Autodesk Inventor part; units mm, degrees
ref_plane "YZ Plane" through (0, 0, 0) normal (1, 0, 0) x (0, 1, 0)
ref_plane "XZ Plane" through (0, 0, 0) normal (0, 1, 0) x (-1, 0, 0)
ref_plane "XY Plane" through (0, 0, 0) normal (0, 0, 1) x (1, 0, 0)
sketch "スケッチ1" plane through (0, 0, 0) normal (0, 0, 1) x (1, 0, 0)
  circle A0 centre (-4.75, 48) radius 1.55
  circle A1 centre (4.75, 48) radius 1.55
  circle A2 centre (-4.75, -48) radius 1.55
  circle A3 centre (4.75, -48) radius 1.55
  line L0 (-4.75, -48) -> (4.75, -48) construction
  line L1 (4.75, -48) -> (4.75, 48) construction
  line L2 (4.75, 48) -> (-4.75, 48) construction
  line L3 (-4.75, 48) -> (-4.75, -48) construction
  line L4 (-4.75, -48) -> (4.75, 48) construction
  line L5 (4.75, -48) -> (-4.75, 48) construction
  line L6 (-17.75, 61) -> (50.25, 61)
  line L7 (50.25, 61) -> (50.25, -104)
  line L8 (50.25, -104) -> (-17.75, -104)
  line L9 (-17.75, -104) -> (-17.75, 61)
  circle A4 centre (44.25, 55) radius 1.55
  line L10 (16.25, 61) -> (16.25, -104) construction
  line L11 (16.25, -21.5) -> (50.25, -21.5) construction
  circle A5 centre (21.25, 55) radius 1.55
  circle A6 centre (33.25, 55) radius 1.55
  line L12 (16.25, 19.75) -> (50.25, 19.75) construction
  line L13 (16.25, 40.375) -> (50.25, 40.375) construction
  circle A7 centre (44.25, 25.75) radius 1.55
  circle A8 centre (44.25, -15.5) radius 1.55
  circle A9 centre (44.25, 13.75) radius 1.55
  circle A10 centre (44.25, -98) radius 1.55
  circle A11 centre (21.25, -98) radius 1.55
  circle A12 centre (33.25, -98) radius 1.55
  circle A13 centre (44.25, -68.75) radius 1.55
  circle A14 centre (44.25, -27.5) radius 1.55
  circle A15 centre (44.25, -56.75) radius 1.55
  circle A16 centre (-11.75, 55) radius 1.55
  circle A17 centre (11.25, 55) radius 1.55
  circle A18 centre (-0.75, 55) radius 1.55
  circle A19 centre (-11.75, 25.75) radius 1.55
  circle A20 centre (-11.75, -15.5) radius 1.55
  circle A21 centre (-11.75, 13.75) radius 1.55
  circle A22 centre (-11.75, -27.5) radius 1.55
  circle A23 centre (-11.75, -56.75) radius 1.55
  circle A24 centre (11.25, -98) radius 1.55
  circle A25 centre (-0.75, -98) radius 1.55
  circle A26 centre (-11.75, -98) radius 1.55
  circle A27 centre (-11.75, -68.75) radius 1.55
  circle A28 centre (-4.75, 38) radius 1.55
  circle A29 centre (4.75, 38) radius 1.55
  circle A30 centre (-4.75, -58) radius 1.55
  circle A31 centre (4.75, -58) radius 1.55
  circle A32 centre (-4.75, 28) radius 1.55
  circle A33 centre (4.75, 28) radius 1.55
  circle A34 centre (-4.75, -68) radius 1.55
  circle A35 centre (4.75, -68) radius 1.55
  circle A36 centre (-4.75, 18) radius 1.55
  circle A37 centre (4.75, 18) radius 1.55
  circle A38 centre (-4.75, -78) radius 1.55
  circle A39 centre (4.75, -78) radius 1.55
  circle A40 centre (-4.75, 8) radius 1.55
  circle A41 centre (4.75, 8) radius 1.55
  circle A42 centre (-4.75, -88) radius 1.55
  circle A43 centre (4.75, -88) radius 1.55
  circle A44 centre (25.5, 36.25) radius 10.75
  line L14 (14.75, 47) -> (36.25, 47) construction
  line L15 (36.25, 47) -> (36.25, -90) construction
  line L16 (36.25, -90) -> (14.75, -90) construction
  line L17 (14.75, -90) -> (14.75, 47) construction
  circle A45 centre (25.5, -0.75) radius 10.75
  circle A46 centre (25.5, -37.75) radius 10.75
  circle A47 centre (25.5, -74.75) radius 10.75
  circle A48 centre (4.75, 48) radius 2.75 construction
  point P0 (0, 0)
  dimension "d0" = 3.1
  dimension "d1" = 9.5
  dimension "d2" = 96
  dimension "d3" = 13
  dimension "d4" = 13
  dimension "d7" = 165
  dimension "d8" = 68
  dimension "d16" = 3.1
  dimension "d17" = 6
  dimension "d18" = 6
  dimension "d19" = 5
  dimension "d20" = 17
  dimension "d21" = 41.25
  dimension "d22" = 20.625
  dimension "d25" = 10
  dimension "d30" = 10
  dimension "d31" = 8
  dimension "d32" = 8
  dimension "d35" = 37
  dimension "d40" = 8
  dimension "d41" = 5.5
extrude "押し出し1" add sketch "スケッチ1" along normal blind 2
equation "\"d1\" = d20_1"
equation "\"d4\" = d3"
equation "\"d8\" = 足_短辺"
equation "\"d18\" = d17"
equation "\"d20\" = 0.25 * d8"
equation "\"d21\" = 0.25 * d7"
equation "\"d22\" = 0.5 * d21"
equation "\"d31\" = d32"
equation "\"d40\" = d31"
equation "\"H_head\" = 96"
equation "\"H_leg\" = 306"
equation "\"足の面積\" = 12720.125"
equation "\"現在の面積\" = 11560"
equation "\"足_短辺\" = 68"
equation "\"円柱\" = 313.5"
equation "\"胴体中心から手先\" = 342"
equation "\"H_leg_1\" = 186.2"
equation "\"H_leg_MAX\" = 399"
equation "\"H_head_1\" = 26.6"
equation "\"H_head_MAX\" = 142.5"
properties part number "足裏_メインフレーム_1_3" material "GFRP"
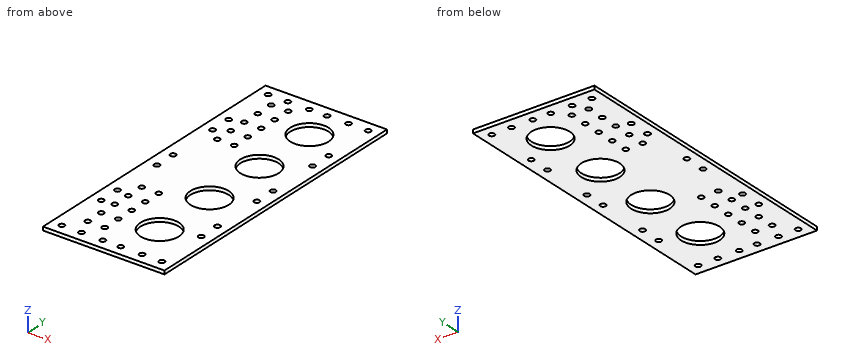
Build history of the part. All positions in model axes, mm. Give positions to 0.01 mm unless a question says otherwise; leave off trailing zeros. Loops run counter-clockwise (first coordinate to the right, second up) from the corner with the lowest first, then second, coordinate; pieces in that order, holes last. Notation, with made-up numbers: (23.25, 39.5) -> (57.25, 39.5) arc R22 cw to (57.25, 57.5) -> close; hole circle Ø3 at (5, 17.25). An arc over 180 degrees is marked (long way). One line per question, with ' | ' between items. Start each with the question number.
1) Cut at D-D (y = -0.75). Give the cut face in (x, z), plus the area to 3 significant figures.
2) Cut at C-C (x = 25.5). Give the cut face in (y, z), plus the area to 3 significant figures.
3) Cut at B-B (y = -98). Give the cut face in (x, z).
4) Cut at A-A (x = -0.75). Give the cut face in (y, z), plus the area to 3 significant figures.
5) Probe L1, parallel to X at y = -56, z = 1.6; L2, parallel to Y at x = 0, z = 0.9; L3, parallel to Y at x = 0.5, z = 1.75. List the from-to ranges inside material, lowest first.
6) Pin check, flat tips, straight feed: pin 1 (1.9 mm diameter, centred on x = 44.25, y = -98, fed in from +Z); pin 2 (5 mm diameter, centred on x = -11.75, y = -27.5, fed in from +Z). Stop position of each tip, or through.
Return value:
1) outline: (-17.75, 0) -> (14.75, 0) -> (14.75, 2) -> (-17.75, 2) -> close; (36.25, 0) -> (50.25, 0) -> (50.25, 2) -> (36.25, 2) -> close | area: 93.0 mm^2
2) outline: (-104, 0) -> (-85.5, 0) -> (-85.5, 2) -> (-104, 2) -> close; (-64, 0) -> (-48.5, 0) -> (-48.5, 2) -> (-64, 2) -> close; (-27, 0) -> (-11.5, 0) -> (-11.5, 2) -> (-27, 2) -> close; (10, 0) -> (25.5, 0) -> (25.5, 2) -> (10, 2) -> close; (47, 0) -> (61, 0) -> (61, 2) -> (47, 2) -> close | area: 158 mm^2
3) outline: (-17.75, 0) -> (-13.3, 0) -> (-13.3, 2) -> (-17.75, 2) -> close; (-10.2, 0) -> (-2.3, 0) -> (-2.3, 2) -> (-10.2, 2) -> close; (0.8, 0) -> (9.7, 0) -> (9.7, 2) -> (0.8, 2) -> close; (12.8, 0) -> (19.7, 0) -> (19.7, 2) -> (12.8, 2) -> close; (22.8, 0) -> (31.7, 0) -> (31.7, 2) -> (22.8, 2) -> close; (34.8, 0) -> (42.7, 0) -> (42.7, 2) -> (34.8, 2) -> close; (45.8, 0) -> (50.25, 0) -> (50.25, 2) -> (45.8, 2) -> close
4) outline: (-104, 0) -> (-99.55, 0) -> (-99.55, 2) -> (-104, 2) -> close; (-96.45, 0) -> (53.45, 0) -> (53.45, 2) -> (-96.45, 2) -> close; (56.55, 0) -> (61, 0) -> (61, 2) -> (56.55, 2) -> close | area: 318 mm^2
5) L1: -17.75 to -13.11, -10.39 to 42.89, 45.61 to 50.25 | L2: -104 to -99.36, -96.64 to 53.64, 56.36 to 61 | L3: -104 to -98.92, -97.08 to 54.08, 55.92 to 61
6) pin 1: through | pin 2: z = 2
